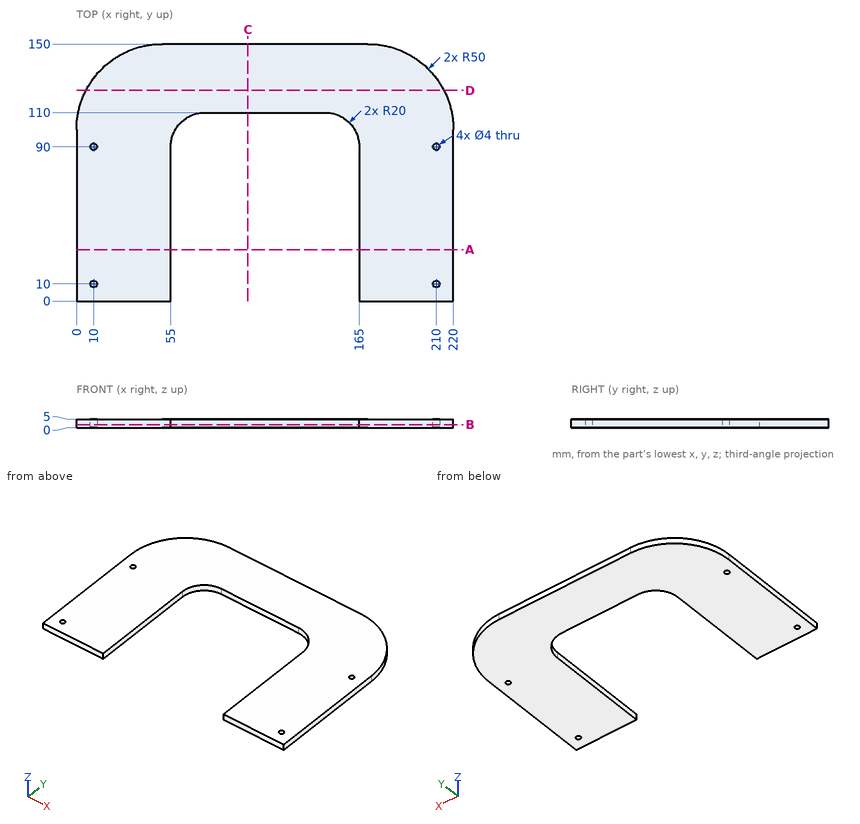
Verification items for this drawing (mm, ordinates from the low corner). Coordinates: 2 decimals unless noted, no trailing zeros. Write each loop counter-clockwise with the first axis right and the second up, starting at its lowest first coordinate (ties: lowest second). Pieces come first, ordered by that corner, then holes. Notation, with made-up numbers: M 89.5,43 L 106.5,43 A8 cw 106.5,54 Z; hole C 51,85.5 d1. An arc over 180 degrees is marked long. Use CSV: the item, a comma, the result in double quotes.
Q1. Section check D-D, the plane y = 123. Enter the section's corners in (x, z).
Computed values:
outline,"M 5.6,0 L 214.4,0 L 214.4,5 L 5.6,5 Z"
Q2. Section check C-C, the plane x = 100. Enter the section's corners in (y, z).
Computed values:
outline,"M 110,0 L 150,0 L 150,5 L 110,5 Z"
Q3. Go/stop test with flat-tipped pins: P1, Ø2, axis at y = 108, z = 0.5, coming from the +X side; P2, Ø4.5, axis at x = 210, y = 10, coming from the +Z side. Record where each tip stops, or that it passes through.
Computed values:
P1,"x = 219.51"
P2,"z = 5"
Q4. Section check A-A, the plane y = 30. Enter the section's corners in (x, z), and give its area (3 significant figures).
Computed values:
outline,"M 0,0 L 55,0 L 55,5 L 0,5 Z; M 165,0 L 220,0 L 220,5 L 165,5 Z"
area,"550 mm²"
Q5. Section check B-B, the plane z = 1.8. Enter the section's corners in (x, y).
Computed values:
outline,"M 0,0 L 55,0 L 55,90 A20 cw 75,110 L 145,110 A20 cw 165,90 L 165,0 L 220,0 L 220,100 A50 ccw 170,150 L 50,150 A50 ccw 0,100 Z; hole C 10,10 d4; hole C 10,90 d4; hole C 210,10 d4; hole C 210,90 d4"
Q6. Thickness scan on line 1 along X through (y, z) = (24, 2.95); line 2 along X through (y, z) = (9, 1.6); line 3 along Y through (x, z) = (90, 3.25). Record the ranges inside material, lowest first. Write a range as [from, to].
Computed values:
line 1,"[0, 55], [165, 220]"
line 2,"[0, 8.27], [11.73, 55], [165, 208.27], [211.73, 220]"
line 3,"[110, 150]"
